Check sheet for the modelled part. Datum: model origin and axes. Units: mm. A direction names the side the tool comes from. Round coordinates to 2 decimals unless told otherwise and drop trailing zeros. Loops run counter-clockwise (first coordinate to the right, second up) from the corner with the lowest first, then second, coordinate; pieces in that order, holes last. Notation, with made-up numbers: (71.5, 30.25) -> (76.5, 30.25) arc R18 cw to (76.5, 63.25) -> close; hole circle Ø3 at (60.5, -12). An arc over 180 degrees is marked (long way). One line per item, written item: value. Start each with the question number.
1. Cross-section at B-B on x = 86.5. Record the cut outline in (y, z) (3 decimals), then the cut area to 3 significant figures.
2. Set-up check for faces 4 (the face through (85, -33, 38.1)), 5 (the face through (-1, -33, -9.525)), 6 (the face through (45.8, -33.1, 38.1)): record each of +Z, -Z, +X, -X, +Y, -Y from which the full face is reachable in a straight line by a thin tool's end or side.
3. Material ranges on L1, parallel to Z at x = 79.5, y = -108 (3 decimals); L2, parallel to X at y = -18.5, z = 5.5 (3 decimals); L3, parallel to X at y = 23.5, z = 25 (3 decimals), recorded low to high.
4. Cross-section at A-A on z = 6.5. Record the cut outline in (x, y) (3 decimals).
5. Release check for a two-part mould opening along X. For faces 1 (the face through (17, 63.5, 29)), 2 (the face through (41.275, -33, 8)), 3 (the face through (60.325, -33, 41)) record: +X half, -X half, draft (parallel to the pull), parting line (faces both ways), or undercut.
6. Go/stop test with flat-tipped pins: pin 1 (8 mm diameter, centred on y = -46.5, z = 27, fed in from +X); pin 2 (6 mm diameter, centred on y = -91, z = 36.5, fed in from -X); pin 3 (1.4 mm diameter, centred on y = -48.5, z = 41, fed in from -X). Record where each tip stops, or that it passes through.
from build123d import *

# Parameters (mm, degrees)
F0_W     = 25.4
F0_H     = 4.7498
F1_DEPTH = 63.5
F2_DEPTH = 63.5


with BuildPart() as f1:
    # F0 (on Front) → F1 (new body, symmetric)
    with BuildSketch(Plane.XZ):
        Polygon((41.275, -9.525), (41.275, 9.525), (22.225, 9.525), (-41.275, 9.525), (-41.275, -9.525), align=None)
        with BuildLine():
            Line((22.225, 9.525), (41.275, 9.525))
            Line((41.275, 9.525), (41.275, 27.0002))
            ThreePointArc((41.275, 27.0002), (45.92468, 38.22552), (57.15, 42.8752))
            Line((57.15, 42.8752), (60.325, 42.8752))
            Line((60.325, 42.8752), (60.325, 61.9252))
            Line((60.325, 61.9252), (57.15, 61.9252))
            ThreePointArc((57.15, 61.9252), (32.454296, 51.695904), (22.225, 27.0002))
            Line((22.225, 27.0002), (22.225, 9.525))
        make_face()
        with BuildLine():
            Line((-41.275, 9.525), (22.225, 9.525))
            Line((22.225, 9.525), (22.225, 27.0002))
            ThreePointArc((22.225, 27.0002), (32.454296, 51.695904), (57.15, 61.9252))
            add(Edge.make_bspline(
                [(-41.275, 9.525), (-39.657938, 44.64065), (26.937186, 65.652682), (57.15, 61.9252)],
                knots=[0, 0, 0, 0, 111.504536, 111.504536, 111.504536, 111.504536], degree=3))
        make_face()
        Polygon((60.325, 61.9252), (60.325, 42.8752), (60.325, 38.1), (111.125, 38.1), (111.125, 66.675), (85.725, 66.675), (85.725, 61.9252), align=None)
        with Locations((73.025, 64.3001)):
            Rectangle(F0_W, F0_H)
    extrude(amount=F1_DEPTH, both=True)

    # F1_face (on face) → F2 (join, symmetric)
    with BuildSketch(Plane(origin=(25.424226, -63.5, 29.456982), x_dir=(1, 0, 0), z_dir=(0, -1, 0))):
        with BuildLine():
            Line((15.850774, -38.981982), (15.850774, -2.456782))
            ThreePointArc((15.850774, -2.456782), (20.500454, 8.768538), (31.725774, 13.418218))
            Line((31.725774, 13.418218), (34.900774, 13.418218))
            Line((34.900774, 13.418218), (34.900774, 8.643018))
            Line((34.900774, 8.643018), (85.700774, 8.643018))
            Line((85.700774, 8.643018), (85.700774, 37.218018))
            Line((85.700774, 37.218018), (34.900774, 37.218018))
            Line((34.900774, 37.218018), (34.900774, 32.468218))
            Line((34.900774, 32.468218), (31.725774, 32.468218))
            add(Edge.make_bspline(
                [(-66.699226, -19.931982), (-65.082164, 15.183668), (1.51296, 36.1957), (31.725774, 32.468218)],
                knots=[0, 0, 0, 0, 111.504536, 111.504536, 111.504536, 111.504536], degree=3))
            Line((-66.699226, -19.931982), (-66.699226, -38.981982))
            Line((-66.699226, -38.981982), (15.850774, -38.981982))
        make_face()
    extrude(amount=F2_DEPTH, both=True)


solid = f1.part
Taken from the geometry:
1. outline: (-127, 38.1) -> (63.5, 38.1) -> (63.5, 66.675) -> (-127, 66.675) -> close
1. area: 5,440 mm2
2. face 4: -Z, +X, +Y, -Y
2. face 5: -Z, +X, -X, +Y, -Y
2. face 6: -Z, +Y, -Y
3. L1: z = 38.1 to 66.675
3. L2: x = -41.275 to 41.275
3. L3: x = -36.088 to 41.275
4. outline: (-41.275, -127) -> (41.275, -127) -> (41.275, 63.5) -> (-41.275, 63.5) -> close
5. face 1: draft
5. face 2: +X half
5. face 3: undercut
6. pin 1: stops at x = 41.79
6. pin 2: stops at x = -29
6. pin 3: stops at x = -20.7
